```python
from build123d import *

# Parameters (mm, degrees)
SKETCH1_W           = 40
SKETCH1_H           = 40
BOSS_EXTRUDE1_DEPTH = 5
SKETCH2_W           = 5
SKETCH2_H           = 40
BOSS_EXTRUDE4_DEPTH = 45
SKETCH6_R           = 6
CUT_EXTRUDE5_DEPTH  = 61.415229868
SKETCH7_R           = 1.5
CUT_EXTRUDE6_DEPTH  = 58.445626465


with BuildPart() as part:
    # Sketch1 → Boss-Extrude1 (new body)
    with BuildSketch(Plane(origin=(0, 0, 0), x_dir=(1, 0, 0), z_dir=(0, 1, 0))):
        Rectangle(SKETCH1_W, SKETCH1_H)
    extrude(amount=BOSS_EXTRUDE1_DEPTH)

    # Sketch2 → Boss-Extrude4 (add)
    with BuildSketch(Plane.XZ):
        with Locations((-17.5, 0)):
            Rectangle(SKETCH2_W, SKETCH2_H)
    extrude(amount=BOSS_EXTRUDE4_DEPTH)

    # Sketch6 → Cut-Extrude5 (cut, through all)
    with BuildSketch(Plane(origin=(-15, 0, 0), x_dir=(0, 0, -1), z_dir=(1, 0, 0))):
        with Locations((0, -36)):
            Circle(SKETCH6_R)
    extrude(amount=-CUT_EXTRUDE5_DEPTH, mode=Mode.SUBTRACT)

    # Sketch7 → Cut-Extrude6 (cut, through all)
    with BuildSketch(Plane(origin=(0, 5, 0), x_dir=(1, 0, 0), z_dir=(0, 1, 0))):
        with Locations(Location((-11.456996051, 17, 0), (0, 0, 270))):
            Circle(SKETCH7_R)
        with Locations(Location((11.456996051, 17, 0), (0, 0, 270))):
            Circle(SKETCH7_R)
        with Locations(Location((11.456996051, -17, 0), (0, 0, 270))):
            Circle(SKETCH7_R)
        with Locations(Location((-11.456996051, -17, 0), (0, 0, 270))):
            Circle(SKETCH7_R)
    extrude(amount=-CUT_EXTRUDE6_DEPTH, mode=Mode.SUBTRACT)


solid = part.part
```
Check sheet for the modelled part. Datum: model origin and axes. Units: mm. A direction names the side the tool comes from. Give positions to 0.01 mm unless a question says otherwise; leave off trailing zeros. Write each loop counter-clockwise with the first axis right and the second up, starting at its lowest first coordinate (ties: lowest second). Pieces come first, ordered by that corner, then holes.
Item 1: Gauge pin test, flat ends, axial feed: pin 1 (12 mm diameter, centred on x = -7.5, z = -5, fed in from -Y); pin 2 (12 mm diameter, centred on y = -23.5, z = -6.5, fed in from +X); pin 3 (4 mm diameter, centred on x = -11.46, z = 17, fed in from +Y). Record the tip position at first contact, or that the pin passes through.
Item 2: Scan lines: L1, parallel to X at y = 2, z = -17; L2, parallel to Y at x = -16.85, z = 0; L3, parallel to Y at x = 18, z = 15.5. Record each from-to range of solid material in increasing order.
Item 3: Cross-section at A-A (z = 17). Enter the section's corners in (x, y).
Item 4: Draft check along X on faces 1 (the face through (-20, -20, 0)), 2 (the face through (-11.4, 2.5, 15.5)), 3 (the face through (2, 0, 0)). Enter one of: released by +X, released by -X, zero draft, split by the parting line, or undercut.
Item 5: Cross-section at C-C (z = 0). Enter the section's corners in (x, y), and give its area (3 significant figures).
Item 6: Cross-section at B-B (y = -36). Enter the section's corners in (x, z).
Item 7: Access from +Z, -Z, +X, -X, +Y, -Y to the whole of each face (thin tool, end or side, straight path). Record for faces 4 (the face through (-11.4, 2.5, -18.5)), 5 (the face through (-15, -22, 0)).
Item 8: Cross-section at D-D (z = -4). Enter the section's corners in (x, y), and give its area (3 significant figures).
Report:
1. pin 1: stops at y = 0
1. pin 2: stops at x = -15
1. pin 3: stops at y = 5
2. L1: x = -20 to -12.96, -9.96 to 9.96, 12.96 to 20
2. L2: y = -45 to -42, -30 to 5
2. L3: y = 0 to 5
3. outline: (-20, -45) - (-15, -45) - (-15, 0) - (-12.96, 0) - (-12.96, 5) - (-20, 5) - close; (-9.96, 0) - (9.96, 0) - (9.96, 5) - (-9.96, 5) - close; (12.96, 0) - (20, 0) - (20, 5) - (12.96, 5) - close
4. face 1: released by -X
4. face 2: undercut
4. face 3: zero draft
5. outline: (-20, -45) - (-15, -45) - (-15, -42) - (-20, -42) - close; (-20, -30) - (-15, -30) - (-15, 0) - (20, 0) - (20, 5) - (-20, 5) - close
5. area: 365 mm2
6. outline: (-20, -20) - (-15, -20) - (-15, -6) - (-20, -6) - close; (-20, 6) - (-15, 6) - (-15, 20) - (-20, 20) - close
7. face 4: +Y, -Y
7. face 5: +Z, -Z, +X, -Y
8. outline: (-20, -45) - (-15, -45) - (-15, -40.47) - (-20, -40.47) - close; (-20, -31.53) - (-15, -31.53) - (-15, 0) - (20, 0) - (20, 5) - (-20, 5) - close
8. area: 380 mm2
